The listing builds one solid part. Answer for the finished solid, in the listing's coordinates (mm). Face numbers are marked on the shaded views. A direction names the side the tool comes from. Coordinates: 2 decimals unless noted, no trailing zeros. Loops run counter-clockwise (first coordinate to the right, second up) from the corner with the lowest first, then second, coordinate; pieces in that order, holes last. Notation, with made-up numbers: M 58.5,19 L 105.5,19 A13 ccw 105.5,42 Z; hole C -2.5,-23.75 d5. An arc over 180 degrees is marked long. Answer as a JSON object with one key per item and string values. Group by question number.
1. A cutting plane is placed at A-A on x = -7. Give the vertices of the cut face in (y, z), and give its area (3 significant figures).
2. Given pin 1 (2.5 mm diameter, centred on x = 7, z = 6.5, fed in from +Y); pin 2 (1.2 mm diameter, centred on x = -5.5, y = 29.5, fed in from +Z); pin 3 (2.5 mm diameter, centred on x = -7, y = 2, fed in from -Z); pin 4 (1.8 mm diameter, centred on x = -7, y = 29, fed in from +Z), each flat-ended and moving along its own axis, determine where each tip first touches the part or whether it passes through.
3. Determine the mould class of the marked faces 1, 2 and 3 for opening direction Y: released by +Y, released by -Y, zero draft, split by the parting line, or undercut.
4. For the marked faces 4 and 5, determine the directions among +Z, -Z, +X, -X, +Y, -Y from which every point of the face is accessible in a straight line to the end or side of a thin tool.
5. A cutting plane is placed at C-C on x = -2. Give the vertices of the cut face in (y, z), and give its area (3 significant figures).
6. Straight lines are drawn through the part: L1, parallel to X at y = 29, z = -2; L2, parallel to X at y = 8, z = 4; L3, parallel to Y at x = -7, z = -1.75. For each, find the intervals that lie inside material, in ascending order.
7. A cutting plane is placed at B-B on y = 29. Give the vertices of the cut face in (x, z), and give its area (3 significant figures).
8. A cutting plane is placed at D-D on z = -6. Give the vertices of the cut face in (x, y).
from build123d import *

# Parameters (mm, degrees)
SKETCH1_W           = 20
SKETCH1_H           = 20
SKETCH1_R           = 2.5
BOSS_EXTRUDE1_DEPTH = 2
SKETCH2_W           = 20
SKETCH2_H           = 20
SKETCH2_R           = 4.5
BOSS_EXTRUDE2_DEPTH = 2
SKETCH6_W           = 3
SKETCH6_H           = 20
BOSS_EXTRUDE4_DEPTH = 4
SKETCH4_W           = 20
SKETCH4_H           = 27
BOSS_EXTRUDE3_DEPTH = 2
SKETCH5_R           = 1
CUT_EXTRUDE1_DEPTH  = 20
SKETCH7_W           = 13.5
SKETCH7_H           = 12
BOSS_EXTRUDE5_DEPTH = 4
FILLET3_R           = 10
SKETCH9_W           = 35
SKETCH9_H           = 31
BOSS_EXTRUDE6_DEPTH = 2


with BuildPart() as part:
    # Sketch1 → Boss-Extrude1 (new body)
    with BuildSketch(Plane(origin=(0, 0, 0), x_dir=(1, 0, 0), z_dir=(0, 1, 0))):
        Rectangle(SKETCH1_W, SKETCH1_H)
        with Locations(Location((4.696699141, -4.696699141, 0), (0, 0, 90))):
            Circle(SKETCH1_R, mode=Mode.SUBTRACT)
        with Locations(Location((4.696699141, 4.696699141, 0), (0, 0, 90))):
            Circle(SKETCH1_R, mode=Mode.SUBTRACT)
    extrude(amount=BOSS_EXTRUDE1_DEPTH)

    # Sketch2 → Boss-Extrude2 (add)
    with BuildSketch(Plane(origin=(0, 2, 0), x_dir=(1, 0, 0), z_dir=(0, 1, 0))):
        Rectangle(SKETCH2_W, SKETCH2_H)
        with Locations(Location((4.696699141, -4.696699141, 0), (0, 0, 270))):
            Circle(SKETCH2_R, mode=Mode.SUBTRACT)
        with Locations(Location((4.696699141, 4.696699141, 0), (0, 0, 270))):
            Circle(SKETCH2_R, mode=Mode.SUBTRACT)
    extrude(amount=BOSS_EXTRUDE2_DEPTH)

    # Sketch6 → Boss-Extrude4 (add)
    with BuildSketch(Plane(origin=(0, 4, 0), x_dir=(1, 0, 0), z_dir=(0, 1, 0))):
        with Locations((-11.5, 0)):
            Rectangle(SKETCH6_W, SKETCH6_H)
    extrude(amount=-BOSS_EXTRUDE4_DEPTH)

    # Sketch4 → Boss-Extrude3 (add)
    with BuildSketch(Plane.ZY.offset(13)):
        with Locations((0, 13.5)):
            Rectangle(SKETCH4_W, SKETCH4_H)
    extrude(amount=BOSS_EXTRUDE3_DEPTH)

    # Sketch5 → Cut-Extrude1 (cut)
    with BuildSketch(Plane(origin=(0, 0, -10), x_dir=(-1, 0, 0), z_dir=(0, 0, -1))):
        with Locations((7, 2)):
            Circle(SKETCH5_R)
    cut_extrude1 = extrude(amount=-CUT_EXTRUDE1_DEPTH, mode=Mode.SUBTRACT)

    # Sketch7 → Boss-Extrude5 (add)
    with BuildSketch(Plane(origin=(0, 27, 0), x_dir=(1, 0, 0), z_dir=(0, 1, 0))):
        with Locations((-8.25, 4)):
            Rectangle(SKETCH7_W, SKETCH7_H)
    extrude(amount=BOSS_EXTRUDE5_DEPTH)

    # Mirror1: Cut-Extrude1 across plane
    add(cut_extrude1.mirror(Plane.ZX.offset(15.5)), mode=Mode.SUBTRACT)

    # Fillet3
    # the kernel refuses this fillet: 10 mm, written as the material it adds along each edge
    with BuildSketch(Plane(origin=(-13, 27, 2), x_dir=(0, 0, 1), z_dir=(-1, 0, 0))) as fillet3_piece_1:
        with BuildLine():
            CenterArc((8, 10), FILLET3_R, 216.869897646, 53.130102354)
            Line((0, 4), (0, 0))
            Line((0, 0), (8, 0))
        make_face()
    extrude(amount=2)

    # Sketch9 → Boss-Extrude6 (add)
    with BuildSketch(Plane(origin=(10, 0, 0), x_dir=(0, 0, -1), z_dir=(1, 0, 0))):
        with Locations((7.5, 15.5)):
            Rectangle(SKETCH9_W, SKETCH9_H)
    extrude(amount=BOSS_EXTRUDE6_DEPTH)


solid = part.part
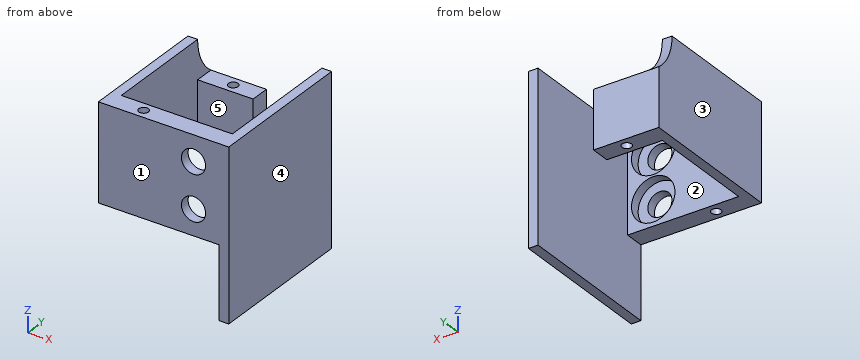
From the geometry:
{
 "1": {"outline": "M 0,-10 L 1,-10 L 1,10 L 0,10 Z; M 3,-10 L 4,-10 L 4,10 L 3,10 Z; M 27,-10 L 28,-10 L 28,2 L 27,2 Z; M 30,-10 L 31,-10 L 31,2 L 30,2 Z", "area": "64.0 mm²"},
 "2": {"pin 1": "stops at y = 2", "pin 2": "stops at z = 2", "pin 3": "stops at z = -10", "pin 4": "passes through"},
 "3": {"face 1": "released by -Y", "face 2": "undercut", "face 3": "zero draft"},
 "4": {"face 4": "+Z, -Z, +X, +Y, -Y", "face 5": "+Z, -Z"},
 "5": {"outline": "M 0,-10 L 4,-10 L 4,10 L 0,10 Z; M 27,-10 L 31,-10 L 31,2 L 27,2 Z", "area": "128 mm²"},
 "6": {"L1": "x = -15 to -8, -6 to -1.5, 10 to 12", "L2": "x = -15 to -13, 10 to 12", "L3": "y = 0 to 1, 3 to 4, 27 to 28, 30 to 31"},
 "7": {"outline": "M -15,-10 L -8,-10 L -8,2 L -13,2 L -13,4 L -15,4 Z; M -6,-10 L -1.5,-10 L -1.5,2 L -6,2 Z; M 10,-25 L 12,-25 L 12,10 L 10,10 Z", "area": "212 mm²"},
 "8": {"outline": "M -15,0 L 2.56,0 L 2.56,2 L 0.39,2 L 0.39,4 L -13,4 L -13,27 L -1.5,27 L -1.5,31 L -15,31 Z; M 6.83,0 L 12,0 L 12,31 L 10,31 L 10,4 L 9,4 L 9,2 L 6.83,2 Z; hole C -7,2 d2; hole C -7,29 d2"}
}
